```python
from build123d import *

# Parameters (mm, degrees)
SKETCH1_W           = 8.9
SKETCH1_H           = 40
BOSS_EXTRUDE1_DEPTH = 29.39
SKETCH5_W           = 27.9
SKETCH5_H           = 23.3
CUT_EXTRUDE2_DEPTH  = 37.646720181
SKETCH7_R           = 1
SKETCH7_R_2         = 11
CUT_EXTRUDE3_DEPTH  = 37.646720181
SKETCH8_W           = 40
SKETCH8_H           = 23.3
CUT_EXTRUDE4_DEPTH  = 37.646720181
SKETCH9_W           = 40
SKETCH9_H           = 2.09
CUT_EXTRUDE5_DEPTH  = 37.646720181


with BuildPart() as part:
    # Sketch1 → Boss-Extrude1 (new body)
    with BuildSketch(Plane(origin=(0, 0, 0), x_dir=(1, 0, 0), z_dir=(0, 1, 0))):
        Rectangle(SKETCH1_W, SKETCH1_H)
    extrude(amount=BOSS_EXTRUDE1_DEPTH)

    # Sketch5 → Cut-Extrude2 (cut, through all)
    with BuildSketch(Plane.ZY.offset(4.45)):
        with Locations((0, 11.65)):
            Rectangle(SKETCH5_W, SKETCH5_H)
    extrude(amount=-CUT_EXTRUDE2_DEPTH, mode=Mode.SUBTRACT)

    # Sketch7 → Cut-Extrude3 (cut, through all)
    with BuildSketch(Plane(origin=(4.45, 0, 0), x_dir=(0, 0, -1), z_dir=(1, 0, 0))):
        with Locations((9.5, 23.3)):
            Circle(SKETCH7_R)
        with Locations((-9.5, 23.3)):
            Circle(SKETCH7_R)
        with Locations((0, 13.8)):
            Circle(SKETCH7_R_2)
    extrude(amount=-CUT_EXTRUDE3_DEPTH, mode=Mode.SUBTRACT)

    # Sketch8 → Cut-Extrude4 (cut, through all)
    with BuildSketch(Plane(origin=(4.45, 0, 0), x_dir=(0, 0, -1), z_dir=(1, 0, 0))):
        with Locations((0, 11.65)):
            Rectangle(SKETCH8_W, SKETCH8_H)
    extrude(amount=-CUT_EXTRUDE4_DEPTH, mode=Mode.SUBTRACT)

    # Sketch9 → Cut-Extrude5 (cut, through all)
    with BuildSketch(Plane(origin=(4.45, 0, 0), x_dir=(0, 0, -1), z_dir=(1, 0, 0))):
        with Locations((0, 28.345)):
            Rectangle(SKETCH9_W, SKETCH9_H)
    extrude(amount=-CUT_EXTRUDE5_DEPTH, mode=Mode.SUBTRACT)


solid = part.part
```
For this review, take the finished solid that the model builds, in its own axes (mm). Round coordinates to 2 decimals unless told otherwise and drop trailing zeros. Write each loop counter-clockwise with the first axis right and the second up, starting at its lowest first coordinate (ties: lowest second). Pieces come first, ordered by that corner, then holes. Notation, with made-up numbers: (13, -6.5) -> (36, -6.5) arc R7 ccw to (36, 3.5) -> close; hole circle Ø6 at (58.25, 43.5). An arc over 180 degrees is marked (long way). One line per question, with ' | ' between items. Start each with the question number.
1) Wall thickness on line 1 along Z through (x, y) = (-2.75, 23.6); line 2 along Z through (x, y) = (-2, 23.95); line 3 along Y through (x, z) = (-1.5, 9): over which ranges is each line inside the solid? List them lowest first.
2) Mouldability with a two-part tool opening along Z and no side actions: class faces 1 (the flat face through (0, 23.3, 7)), 2 (the cylindrical face through (0.1, 24.3, 9.5)), 3 (the flat face through (0, 25, 20)), 4 (the flat face through (0, 25, -20)) as +Z half, -Z half, draft (parallel to the pull), parting line (faces both ways), or undercut.
3) Add section B-B (y = 23.95). Write out the cut boundary in (x, z).
4) Add section C-C (z = 9.5). Write out the cut boundary in (x, y), and give its area (3 significant figures).
5) Add section A-A (x = 0.5). Write out the cut boundary in (y, z), and give its area (3 significant figures).
Reported:
1) line 1: z = -20 to -10.45, -8.55 to -5, 5 to 8.55, 10.45 to 20 | line 2: z = -20 to -10.26, -8.74 to -4.24, 4.24 to 8.74, 10.26 to 20 | line 3: y = 24.17 to 27.3
2) face 1: draft | face 2: undercut | face 3: +Z half | face 4: -Z half
3) outline: (-4.45, -20) -> (4.45, -20) -> (4.45, -10.26) -> (-4.45, -10.26) -> close; (-4.45, -8.74) -> (4.45, -8.74) -> (4.45, -4.24) -> (-4.45, -4.24) -> close; (-4.45, 4.24) -> (4.45, 4.24) -> (4.45, 8.74) -> (-4.45, 8.74) -> close; (-4.45, 10.26) -> (4.45, 10.26) -> (4.45, 20) -> (-4.45, 20) -> close
4) outline: (-4.45, 24.3) -> (4.45, 24.3) -> (4.45, 27.3) -> (-4.45, 27.3) -> close | area: 26.7 mm²
5) outline: (23.3, -20) -> (27.3, -20) -> (27.3, 20) -> (23.3, 20) -> (23.3, 10.5) arc R1 cw to (23.3, 8.5) -> (23.3, 5.55) arc R11 cw to (23.3, -5.55) -> (23.3, -8.5) arc R1 cw to (23.3, -10.5) -> close | area: 146 mm²
